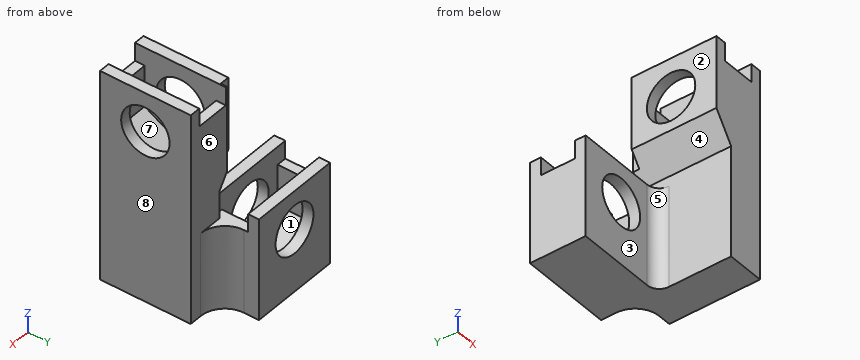
from build123d import *

# Parameters (mm, degrees)
SKETCH046_W       = 7.5
SKETCH046_H       = 8.4
SKETCH046_R       = 2
PAD028_DEPTH      = 4.6
POCKET013_START   = -0.9
POCKET013_DEPTH   = 2.8
PAD029_DEPTH      = 6.15
PAD029_DEPTH_BACK = 1.35
SKETCH049_R       = 2
POCKET014_DEPTH   = 10.551
POCKET015_START   = -0.9
POCKET015_DEPTH   = 2.8
SKETCH051_W       = 0.8
SKETCH051_H       = 0.5
POCKET016_DEPTH   = 8
FILLET008_R       = 1
FILLET009_R       = 2


with BuildPart() as obj1:
    # Sketch046 → Pad028 (new body)
    with BuildSketch(Plane.XZ):
        with Locations((0, -1)):
            Rectangle(SKETCH046_W, SKETCH046_H)
        Circle(SKETCH046_R, mode=Mode.SUBTRACT)
    extrude(amount=PAD028_DEPTH)

    # Sketch047 (on Face7 of Pad028) → Pocket013 (cut)
    with BuildSketch(Plane.XZ.offset(4.6).offset(POCKET013_START)):
        Polygon((2.95, 1.703183), (3.75, 1.703183), (3.75, 3.2), (-3.75, 3.2), (-3.75, 1.703183), (-2.95, 1.703183), (-2.95, -1.703183), (0, -3.406367), (2.95, -1.703183), align=None)
    extrude(amount=-POCKET013_DEPTH, mode=Mode.SUBTRACT)

    # Sketch048 (on Face8 of Pocket013) → Pad029 (join, two sides)
    with BuildSketch(Plane.XZ.offset(4.6)) as pad029_sk:
        Polygon((-3.75, -5.2), (-3.75, 3.2), (-3.75, 4), (-2.2, 6.213629), (-2.2, 12.213629), (-6.8, 12.213629), (-6.8, -5.2), align=None)
    extrude(amount=PAD029_DEPTH)
    extrude(pad029_sk.sketch, amount=-PAD029_DEPTH_BACK)

    # Sketch049 (on Face26 of Pad029) → Pocket014 (cut, through all)
    with BuildSketch(Plane(origin=(-6.8, 0, 0), x_dir=(0, 0, -1), z_dir=(-1, 0, 0))):
        with Locations((-9.003629, 7)):
            Circle(SKETCH049_R)
    extrude(amount=-POCKET014_DEPTH, mode=Mode.SUBTRACT)

    # Sketch050 (on Face26 of Pocket014) → Pocket015 (cut)
    with BuildSketch(Plane(origin=(-6.8, 0, 0), x_dir=(0, 0, -1), z_dir=(-1, 0, 0)).offset(POCKET015_START)):
        Polygon((-10.706813, 9.95), (-10.706813, 10.75), (-12.213629, 10.75), (-12.213629, 3.25), (-10.706813, 3.25), (-10.706813, 4.05), (-7.300446, 4.05), (-5.597263, 7), (-7.300446, 9.95), align=None)
    extrude(amount=-POCKET015_DEPTH, mode=Mode.SUBTRACT)

    # Sketch051 (on Face25 of Pocket015) → Pocket016 (cut)
    with BuildSketch(Plane(origin=(0, 0, 12.213629), x_dir=(-1, 0, 0), z_dir=(0, 0, 1))):
        with Locations((2.6, 3.5)):
            Rectangle(SKETCH051_W, SKETCH051_H)
    extrude(amount=-POCKET016_DEPTH, mode=Mode.SUBTRACT)

    # Fillet008
    fillet008_edges = [obj1.edges().sort_by_distance(p)[0] for p in [
        (-3.75, -4.6, -1),
    ]]
    fillet(fillet008_edges, radius=FILLET008_R)

    # Fillet009
    fillet009_edges = [obj1.edges().sort_by_distance(p)[0] for p in [
        (-3.75, -3.25, -1.748408),
    ]]
    fillet(fillet009_edges, radius=FILLET009_R)


with BuildPart() as obj1_1:
    # Body027 placement: moved
    add(obj1.part.moved(Location((-30, 36.8, 6.9))))


with BuildPart() as part_mirroring:
    # Part__Mirroring: instance of obj1
    add(obj1_1.part.mirror(Plane(origin=(0, 0, 0), x_dir=(0, -1, 0), z_dir=(1, 0, 0))))


solid = part_mirroring.part
Could you check a few things on this model? Use its own coordinates, in mm. Face numbers are marked on the shaded views. A direction names the side the tool comes from. Coordinates: 2 decimals unless noted, no trailing zeros. Write each loop counter-clockwise with the first axis right and the second up, starting at its lowest first coordinate (ties: lowest second). Pieces come first, ordered by that corner, then holes. Notation, with made-up numbers: (36, -37.5) - (54, -37.5) arc R18 ccw to (54, -6.5) - close; hole circle Ø10 at (78.25, 16.25). An arc over 180 degrees is marked (long way). Put each result on its own line as item: value. Start each with the question number.
Q1. I'm going to push flat-ended pins straight in: P1, Ø2, axis at x = 29, y = 32.5, coming from the +Z side; P2, Ø3, axis at x = 34, z = 15.5, coming from the +Y side; P3, Ø0.9, axis at x = 26.5, y = 34.5, coming from the +Z side; P4, Ø3, axis at x = 30, z = 6.9, coming from the +Y side. Where does each tip first touch, or does it pass through?
Q2. Thinking about a two-plate mould opening in X: for the marked faces 1, 2 and 3, which applies, pulls with the +X half, pulls with the -X half, needs draft (parallel to the pull), parting line crosses it, or undercut?
Q3. I want a section at B-B on x = 29.75. Write out the boundary of the cut face in (y, z), plus the area to 3 significant figures.
Q4. I want a section at D-D on z = 17. Write out the boundary of the cut face in (x, y).
Q5. Please list where these lines run through material, in increasing order: L1, parallel to Y at x = 33.25, z = 15.75; L2, parallel to Y at x = 27.75, z = 5.75; L3, parallel to X at y = 32.7, z = 6.9.
Q6. Which directions (+Z, -Z, +X, -X, +Y, -Y) give clear straight access to the entire face, cutting with the end or side of a thin tool? Please do the marked faces 4, 5, 6, 7 and 8.
Q7. I want a section at C-C on y = 27.5. Write out the boundary of the cut face in (x, z).
Q8. I want a section at A-A on z = 6.9. Write out the boundary of the cut face in (x, y).
Checks:
1. P1: z = 10.1
1. P2: y = 33.55
1. P3: z = 8.6
1. P4: through
2. face 1: undercut
2. face 2: pulls with the -X half
2. face 3: needs draft
3. outline: (32.2, 1.7) - (36.8, 1.7) - (36.8, 4.92) - (35.9, 4.92) - (35.9, 3.64) - (33.1, 3.64) - (33.1, 4.92) - (32.2, 4.92) - close; (32.2, 8.88) - (33.1, 8.88) - (33.1, 10.1) - (32.2, 10.1) - close; (35.9, 8.88) - (36.8, 8.88) - (36.8, 10.1) - (35.9, 10.1) - close
3. area: 13.4 mm²
4. outline: (32.2, 26.05) - (36.8, 26.05) - (36.8, 28.13) - (35.9, 28.13) - (35.9, 26.85) - (33.1, 26.85) - (33.1, 28.13) - (32.2, 28.13) - close; (32.2, 31.47) - (33.1, 31.47) - (33.1, 32.75) - (35.9, 32.75) - (35.9, 31.47) - (36.8, 31.47) - (36.8, 33.55) - (33, 33.55) - (33, 33.05) - (32.2, 33.05) - close
5. L1: 26.05 to 26.85, 32.75 to 33.55
5. L2: 32.2 to 33.1, 35.9 to 36.8
5. L3: 26.25 to 28, 32 to 36.8
6. face 4: -X, +Y, -Y
6. face 5: -Z, -X, -Y
6. face 6: +Z, +X, +Y
6. face 7: +Z
6. face 8: +Z, -Z, +X, +Y, -Y
7. outline: (32.2, 13.11) - (33.75, 10.9) - (33.75, 1.7) - (36.8, 1.7) - (36.8, 19.11) - (35.9, 19.11) - (35.9, 13.83) - (33.1, 13.83) - (33.1, 19.11) - (32.2, 19.11) - close
8. outline: (26.25, 32.2) - (28, 32.2) - (28, 33.1) - (27.05, 33.1) - (27.05, 35.9) - (28, 35.9) - (28, 36.8) - (26.25, 36.8) - close; (32, 32.2) - (32.75, 32.2) arc R1 cw to (33.75, 31.2) - (33.75, 26.05) - (36.8, 26.05) - (36.8, 33.55) - (35.75, 33.55) arc R2 cw to (33.75, 35.55) - (33.75, 36.8) - (32, 36.8) - (32, 35.9) - (32.95, 35.9) - (32.95, 33.1) - (32, 33.1) - close
